Model file for the job. Use its own axes, mm. Face numbers are marked on the shaded views. A direction names the side the tool comes from. Coordinates: 2 decimals unless noted, no trailing zeros. Loops run counter-clockwise (first coordinate to the right, second up) from the corner with the lowest first, then second, coordinate; pieces in that order, holes last. Notation, with made-up numbers: M 32.5,60.5 L 74.5,60.5 A19 cw 74.5,97.5 Z; hole C -14.5,41 d11. An arc over 180 degrees is marked long. Write item = value, one per line. Start each with the question number.
from build123d import *

# Parameters (mm, degrees)
SKETCH1_R           = 7.9375
BOSS_EXTRUDE1_DEPTH = 27.10000002
SKETCH2_R           = 3
CUT_EXTRUDE1_DEPTH  = 36.5
SKETCH3_R           = 6
BOSS_EXTRUDE2_DEPTH = 4.64
SKETCH4_R           = 7.9375
BOSS_EXTRUDE3_DEPTH = 4.76
CUT_EXTRUDE2_START  = -81.214
SKETCH5_R           = 3
CUT_EXTRUDE2_DEPTH  = 81.214
SKETCH8_W           = 12.7
SKETCH8_H           = 12.7
BOSS_EXTRUDE5_DEPTH = 8.255
SKETCH11_R          = 3.96875
BOSS_EXTRUDE7_DEPTH = 1.27
SKETCH12_R          = 3.96875
BOSS_EXTRUDE8_DEPTH = 1.778
BOSS_EXTRUDE8_TAPER = 65
SKETCH13_R          = 2.9718
CUT_EXTRUDE9_DEPTH  = 25.4
SKETCH14_R          = 0.02
CUT_EXTRUDE10_DEPTH = 254


with BuildPart() as part:
    # Sketch1 → Boss-Extrude1 (new body)
    with BuildSketch(Plane(origin=(0, 0, 0), x_dir=(1, 0, 0), z_dir=(0, 1, 0))):
        with Locations(Location((0, 0, 0), (0, 0, 270))):
            Circle(SKETCH1_R)
    extrude(amount=BOSS_EXTRUDE1_DEPTH)

    # Sketch2 → Cut-Extrude1 (cut)
    with BuildSketch(Plane(origin=(0, 27.10000002, 0), x_dir=(1, 0, 0), z_dir=(0, 1, 0))):
        with Locations(Location((0, 0, 0), (0, 0, 270))):
            Circle(SKETCH2_R)
    extrude(amount=-CUT_EXTRUDE1_DEPTH, mode=Mode.SUBTRACT)

    # Sketch3 → Boss-Extrude2 (add)
    with BuildSketch(Plane(origin=(0, 27.10000002, 0), x_dir=(1, 0, 0), z_dir=(0, 1, 0))):
        with Locations(Location((0, 0, 0), (0, 0, 270))):
            Circle(SKETCH3_R)
    extrude(amount=BOSS_EXTRUDE2_DEPTH)

    # Sketch4 → Boss-Extrude3 (add)
    with BuildSketch(Plane(origin=(0, 31.74000002, 0), x_dir=(1, 0, 0), z_dir=(0, 1, 0))):
        with Locations(Location((0, 0, 0), (0, 0, 270))):
            Circle(SKETCH4_R)
    extrude(amount=BOSS_EXTRUDE3_DEPTH)

    # Sketch5 → Cut-Extrude2 (cut)
    with BuildSketch(Plane.XZ.offset(CUT_EXTRUDE2_START)):
        with Locations(Location((0, 0, 0), (0, 0, 90))):
            Circle(SKETCH5_R)
    extrude(amount=CUT_EXTRUDE2_DEPTH, mode=Mode.SUBTRACT)

    # Sketch8 → Boss-Extrude5 (add)
    with BuildSketch(Plane.XZ):
        with Locations((2.286, 0)):
            Rectangle(SKETCH8_W, SKETCH8_H)
    extrude(amount=BOSS_EXTRUDE5_DEPTH)

    # Sketch11 → Boss-Extrude7 (add)
    with BuildSketch(Plane.XZ.offset(8.255)):
        with Locations(Location((0, 0, 0), (0, 0, 90))):
            Circle(SKETCH11_R)
    extrude(amount=BOSS_EXTRUDE7_DEPTH)

    # Sketch12 → Boss-Extrude8 (add)
    with BuildSketch(Plane(origin=(0, -9.525, 0), x_dir=(-1, 0, 0), z_dir=(0, -1, 0))):
        with Locations(Location((0, 0, 0), (0, 0, 270))):
            Circle(SKETCH12_R)
    extrude(amount=BOSS_EXTRUDE8_DEPTH, taper=BOSS_EXTRUDE8_TAPER)

    # Sketch13 → Cut-Extrude9 (cut)
    with BuildSketch(Plane(origin=(0, 0, -6.35), x_dir=(-1, 0, 0), z_dir=(0, 0, -1))):
        with Locations((-5.588, -3.888060816)):
            Circle(SKETCH13_R)
    extrude(amount=-CUT_EXTRUDE9_DEPTH, mode=Mode.SUBTRACT)

    # Sketch14 → Cut-Extrude10 (cut)
    with BuildSketch(Plane(origin=(0, 36.50000002, 0), x_dir=(1, 0, 0), z_dir=(0, 1, 0))):
        with Locations(Location((0, 0, 0), (0, 0, 270))):
            Circle(SKETCH14_R)
    extrude(amount=-CUT_EXTRUDE10_DEPTH, mode=Mode.SUBTRACT)


solid = part.part
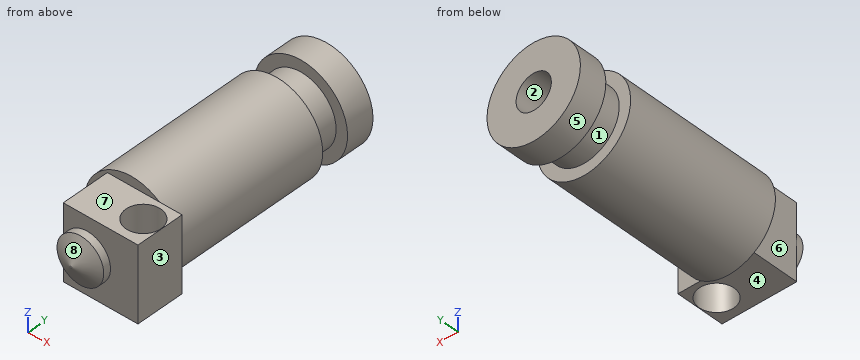
Item 1: Pin check, flat tips, straight feed: pin 1 Ø9 at (x, y) = (4, -3.5) entering from -Z; pin 2 Ø3 at (x, z) = (-0.5, -1) entering from +Y; pin 3 Ø1.5 at (x, y) = (6.5, 17.5) entering from +Z. Stop position of each tip, or through.
Item 2: 3-axis set-ups, long thin cutter, end or side, ignore diameter. For the marked faces 4, 5, 6, 7 and 8: which of +Z, -Z, +X, -X, +Y, -Y reach the whole face in a straight line?
Item 3: Cut at C-C (y = 1). Give the cut face in (x, z) (1 decimal).
Item 4: Cut at B-B (z = 4.5). Give the cut face in (x, y) (3 decimals), plus the area to 3 significant figures.
Item 5: Cut at A-A (x = -5.5). Give the cut face in (y, z), plus the area to 3 significant figures.
Item 6: Pull direction Z, two halves, no side cores. Call the marked faces 1, 2 and 3: +Z half, -Z half, draft (parallel to the pull), parting line (faces both ways), or undercut.
Item 7: Probe L1, parallel to Y at x = -3.25, z = 5.25 (3 decimals); L2, parallel to Z at x = 3.75, y = -8; L3, parallel to Y at x = -5.75, z = 5. List the from-to ranges inside material, lowest first.
Reported:
q1.pin_1 = -7.85
q1.pin_2 = 0
q1.pin_3 = 5.47
q2.face_4 = -Z, +X, -X, -Y
q2.face_5 = +Y
q2.face_6 = +Z, -Z, -X, -Y
q2.face_7 = +Z, +X, -X, -Y
q2.face_8 = -Y
q3.outline = C 0,0 d15.9; hole C 0,0 d6
q4.outline = M -6.539,0 L -4.064,0 L -4.064,-8.255 L 8.636,-8.255 L 8.636,0 L 6.539,0 L 6.539,27.1 L 3.969,27.1 L 3.969,31.74 L 6.539,31.74 L 6.539,36.5 L -6.539,36.5 L -6.539,31.74 L -3.969,31.74 L -3.969,27.1 L -6.539,27.1 Z; hole C 5.588,-3.888 d5.944
q4.area = 531 mm^2
q5.outline = M 0,-5.72 L 27.1,-5.72 L 27.1,-2.4 L 31.74,-2.4 L 31.74,-5.72 L 36.5,-5.72 L 36.5,5.72 L 31.74,5.72 L 31.74,2.4 L 27.1,2.4 L 27.1,5.72 L 0,5.72 Z
q5.area = 387 mm^2
q6.face_1 = parting line
q6.face_2 = undercut
q6.face_3 = draft
q7.L1 = -8.255 to 27.1, 31.74 to 36.5
q7.L2 = -6.35 to 6.35
q7.L3 = 0 to 27.1, 31.74 to 36.5
